Autodesk Inventor part; units mm, degrees
ref_plane "YZ Plane" through (0, 0, 0) normal (1, 0, 0) x (0, 1, 0)
ref_plane "XZ Plane" through (0, 0, 0) normal (0, 1, 0) x (-1, 0, 0)
ref_plane "XY Plane" through (0, 0, 0) normal (0, 0, 1) x (1, 0, 0)
sketch "Sketch1" plane through (0, 0, 0) normal (0, 0, 1) x (1, 0, 0)
  point P0 (0, 0)
sketch "Sketch2" plane through (0, 0, 0) normal (1, 0, 0) x (0, 1, 0)
  circle A0 centre (0, 0) radius 5
  dimension "d0" = 10
extrude "Extrusion1" add sketch "Sketch2" along normal blind 96.4
sketch "Sketch3" plane through (0, 0, 0) normal (-1, 0, 0) x (0, 0, 1)
  circle A0 centre (0, 0) radius 5
  line L0 (-5, 0) -> (5, 0)
  arc A1 (5, 0) -> (-5, 0) centre (0, 0) ccw
  dimension "d3" = 5
extrude "Extrusion2" cut sketch "Sketch3" against normal blind 15 contours L0 A0 picked at (1.2475, 1.1052)
sketch "Sketch4" plane through (0, 0, 5) normal (0, 1, 0) x (1, 0, 0)
  line L0 (15, 0) -> (0, 0)
  line L1 (15, 0) -> (15, 10)
  line L2 (0, 0) -> (15, 0)
  line L3 (15, 0) -> (15, 10)
  line L4 (15, 10) -> (0, 10)
  line L5 (0, 10) -> (0, 0)
  point P0 (0, 5)
extrude "Extrusion3" add sketch "Sketch4" along normal blind 25
sketch "Sketch5" plane through (0, 0, 5) normal (0, 0, 1) x (1, 0, 0)
  line L0 (0, 0) -> (0, 25)
  line L1 (0, 25) -> (15, 25)
  line L2 (15, 25) -> (15, 21)
  line L3 (15, 21) -> (0, 21)
  line L4 (0, 21) -> (0, 25)
  point P0 (0, 21)
  dimension "d8" = 4
  dimension "d9" = 15
extrude "Extrusion4" add sketch "Sketch5" along normal blind 10
sketch "Sketch6" plane through (0, 21, 5) normal (0, -1, 0) x (1, 0, 0)
  circle A0 centre (7.5, 5) radius 3.5
  line L0 (0, 0) -> (0, 10)
  line L1 (15, 0) -> (0, 0)
  point P0 (0, -5)
  dimension "d12" = 7
  dimension "d13" = 7.5
  dimension "d14" = 5
extrude "Extrusion5" cut sketch "Sketch6" against normal blind 2.8
sketch "Sketch7" plane through (7.5, 23.8, 10) normal (0, -1, 0) x (1, 0, 0)
  circle A0 centre (0, 0) radius 2
  line L0 (-7.5, -5) -> (-7.5, 5)
  line L1 (7.5, -5) -> (-7.5, -5)
  point P0 (-7.5, -10)
  dimension "d17" = 7.5
  dimension "d18" = 5
  dimension "d19" = 4
extrude "Extrusion6" cut sketch "Sketch7" against normal through all
mirror "Mirror1" about plane through (96.4, 0, 0) normal (1, 0, 0) of "Extrusion5", "Extrusion6", "Extrusion4", "Extrusion3", "Extrusion1"
properties part number "Supporting-Rod"
Can you work these out from the model? Positions are in its coordinate system, mm. A direction names the side the tool comes from. Give positions to 0.01 mm unless a question says otherwise; leave off trailing zeros. Order: outer loops, then holes, each group sorted by start corner. A loop starts at its lowest first (then second) coordinate and runs counter-clockwise, first axis right, second up. Notation, with made-up numbers: (-29, 72) - (17, 72) arc R24 cw to (17, 98) - close; hole circle Ø1 at (-31, 43). An arc over 180 degrees is marked (long way). Use a Markdown table: item, result. Add a question column.
Q1. I'm going to push flat-ended pins straight in: pin 1 (16.5 mm diameter, centred on x = 183.5, y = 12, fed in from +Z); pin 2 (2 mm diameter, centred on x = 172.5, y = 3.5, fed in from +Z); pin 3 (3 mm diameter, centred on x = 187.5, z = 11.5, fed in from -Y); pin 4 (10 mm diameter, centred on x = 124, z = 11.5, fed in from +Y). Where does each tip first touch, or does it pass through?
Q2. If we section it at B-B on z = 10: Write out the boundary of the cut face in (x, y).
Q3. Please list where these lines run through material, in increasing order: line 1 along Z through (x, y) = (185.3, 24.55); line 2 along X through (y, z) = (21.5, 7); line 3 along Z through (x, y) = (7.5, 22.3).
Q4. On a 3-axis mill with a long thin cutter (end or side, diameter ignored), from which of +Z, -Z, +X, -X, +Y, -Y can I reach the whole of each face in a straight line? I mean faces 1 (the cylindrical face through (6.741, 22.38, 6.583)), 2 (the flat face through (189, 21, 11)), 3 (the cylindrical face through (183.453, 24.392, 10.766)). Say none if no direction works.
Q5. If we section it at C-C on x = 185.3: Write out the boundary of the cut face in (y, z), plus the area to 3 significant figures.
Q6. If we section it at A-A on y = 12.25: Write out the boundary of the cut face in (x, z).
Q7. If we section it at D-D on z = -3: Write out the boundary of the cut face in (x, y), plus the area to 3 significant figures.
Q8. If we mould it in two halves opening along Z, with no side actions, what happens to faces 4 (the flat face through (0, 13, 0)), 5 (the flat face through (9, 23.8, 8)), 6 (the cylindrical face through (98, -5, 0))? For each: released by +Z, released by -Z, zero draft, split by the parting line, or undercut.
Answers follow:
| question | item | result |
|---|---|---|
| 1 | pin 1 | stops at z = 5 |
| 1 | pin 2 | stops at z = 4.33 |
| 1 | pin 3 | stops at y = 21 |
| 1 | pin 4 | passes through |
| 2 | outline | (0, 21) - (4, 21) - (4, 23.8) - (5.5, 23.8) - (5.5, 25) - (0, 25) - close; (9.5, 23.8) - (11, 23.8) - (11, 21) - (15, 21) - (15, 25) - (9.5, 25) - close; (177.8, 21) - (181.8, 21) - (181.8, 23.8) - (183.3, 23.8) - (183.3, 25) - (177.8, 25) - close; (187.3, 23.8) - (188.8, 23.8) - (188.8, 21) - (192.8, 21) - (192.8, 25) - (187.3, 25) - close |
| 3 | line 1 | z = -5 to 8, 12 to 15 |
| 3 | line 2 | x = 0 to 5.7, 9.3 to 15, 177.8 to 183.5, 187.1 to 192.8 |
| 3 | line 3 | z = -5 to 6.5, 13.5 to 15 |
| 4 | face 1 | -Y |
| 4 | face 2 | +Z, +X, -X, -Y |
| 4 | face 3 | +Y, -Y |
| 5 | outline | (0, -5) - (25, -5) - (25, 8) - (23.8, 8) - (23.8, 6.5) - (21, 6.5) - (21, 5) - (0, 5) arc R5 ccw to start; (21, 13.5) - (23.8, 13.5) - (23.8, 12) - (25, 12) - (25, 15) - (21, 15) - close |
| 5 | area | 305 mm^2 |
| 6 | outline | (0, -5) - (15, -5) - (15, 5) - (0, 5) - close; (177.8, -5) - (192.8, -5) - (192.8, 5) - (177.8, 5) - close |
| 7 | outline | (0, -4) - (192.8, -4) - (192.8, 25) - (177.8, 25) - (177.8, 4) - (15, 4) - (15, 25) - (0, 25) - close |
| 7 | area | 2,170 mm^2 |
| 8 | face 4 | zero draft |
| 8 | face 5 | undercut |
| 8 | face 6 | split by the parting line |
